The listing builds one solid part. Answer for the finished solid, in the listing's coordinates (mm). A direction names the side the tool comes from. Round coordinates to 2 decimals unless told otherwise and drop trailing zeros. Write each loop counter-clockwise with the first axis right and the second up, starting at its lowest first coordinate (ties: lowest second). Pieces come first, ordered by that corner, then holes.
from build123d import *

# Parameters (mm, degrees)
SKETCH1_R               = 5
BOSS_EXTRUDE1_DEPTH     = 1
SKETCH2_R               = 3
BOSS_EXTRUDE2_DEPTH     = 12
CHAMFER1_SIZE           = 0.3
CUT_EXTRUDE1_DEPTH      = 15.798648587
CUT_EXTRUDE1_DEPTH_BACK = 15.798648587
SKETCH3_R               = 2.5


with BuildPart() as part:
    # Sketch1 → Boss-Extrude1 (new body)
    with BuildSketch(Plane(origin=(0, 0, 0), x_dir=(1, 0, 0), z_dir=(0, 1, 0))):
        with Locations(Location((0, 0, 0), (0, 0, 270))):
            Circle(SKETCH1_R)
    extrude(amount=BOSS_EXTRUDE1_DEPTH)

    # Sketch2 → Boss-Extrude2 (add)
    with BuildSketch(Plane(origin=(0, 1, 0), x_dir=(1, 0, 0), z_dir=(0, 1, 0))):
        with Locations(Location((0, 0, 0), (0, 0, 270))):
            Circle(SKETCH2_R)
    extrude(amount=BOSS_EXTRUDE2_DEPTH)

    # Chamfer1
    chamfer1_edges = [part.edges().sort_by_distance(p)[0] for p in [
        (0, 13, -3),
    ]]
    chamfer(chamfer1_edges, length=CHAMFER1_SIZE)

    # Sketch3 → Cut-Extrude1 (cut, two sides: drawn at the far end of the back side and taken through both)
    with BuildSketch(Plane(origin=(0, 13, 0), x_dir=(1, 0, 0), z_dir=(0, 1, 0)).offset(-CUT_EXTRUDE1_DEPTH_BACK)):
        with Locations(Location((0, 0, 0), (0, 0, 270))):
            Circle(SKETCH3_R)
    extrude(amount=CUT_EXTRUDE1_DEPTH + CUT_EXTRUDE1_DEPTH_BACK, mode=Mode.SUBTRACT)


solid = part.part
1. A tool of negligible diameter and unlimited length cuts with its end or side. For faces 1 (the face through (-2, 0, 2)), 2 (the face through (0.9, 6.77, 2.86)), from which of +Z, -Z, +X, -X, +Y, -Y can it reach the whole face along a straight path? Write none if from no direction.
Geometry says:
face 1: +Z, -Z, +X, -X, -Y
face 2: +Y
2. Given pin 1 (1.5 mm diameter, centred on y = 11, z = 3.5, fed in from -X); pin 2 (6 mm diameter, centred on y = 9, z = 0.5, fed in from -X); pin 3 (1 mm diameter, centred on y = 6.5, z = -2, fed in from +X), each flat-ended and moving along its own axis, determine where each tip first touches the part or whether it passes through.
Geometry says:
pin 1: stops at x = -1.2
pin 2: stops at x = -3
pin 3: stops at x = 2.6
3. Section B-B on z = 0 is taken. Determine the outline of the cut face in (x, y), plus the area to 3 significant figures.
Geometry says:
outline: (-5, 0) - (-2.5, 0) - (-2.5, 13) - (-2.7, 13) - (-3, 12.7) - (-3, 1) - (-5, 1) - close; (2.5, 0) - (5, 0) - (5, 1) - (3, 1) - (3, 12.7) - (2.7, 13) - (2.5, 13) - close
area: 16.9 mm2
4. Section C-C on y = 4 is taken. Determine the outline of the cut face in (x, z), plus the area to 3 significant figures.
Geometry says:
outline: circle Ø6 at (0, 0); hole circle Ø5 at (0, 0)
area: 8.64 mm2
5. Section D-D on z = -4 is taken. Determine the outline of the cut face in (x, y).
Geometry says:
outline: (-3, 0) - (3, 0) - (3, 1) - (-3, 1) - close
6. For a pull along X with two mould halves and no side action, classify faces 3 (the face through (-3.3, 1, -0.1)), 4 (the face through (-4.88, 0.49, -1.08)), 5 (the face through (-2.44, 6.41, -0.54)) as released by +X, released by -X, zero draft, split by the parting line, or undercut.
Geometry says:
face 3: zero draft
face 4: split by the parting line
face 5: undercut
7. Straight lines are drawn through the part: line 1 along X through (y, z) = (4, 0); line 2 along Y through (x, z) = (-3, -1.25); line 3 along X through (y, z) = (10.5, -1.25). For each, find the intervals that lie inside material, in ascending order.
Geometry says:
line 1: x = -3 to -2.5, 2.5 to 3
line 2: y = 0 to 1
line 3: x = -2.73 to -2.17, 2.17 to 2.73
8. Section A-A on x = 0 is taken. Determine the outline of the cut face in (y, z).
Geometry says:
outline: (0, -5) - (1, -5) - (1, -3) - (12.7, -3) - (13, -2.7) - (13, -2.5) - (0, -2.5) - close; (0, 2.5) - (13, 2.5) - (13, 2.7) - (12.7, 3) - (1, 3) - (1, 5) - (0, 5) - close
